Autodesk Inventor part; units mm, degrees
ref_plane "YZ Plane" through (0, 0, 0) normal (1, 0, 0) x (0, 1, 0)
ref_plane "XZ Plane" through (0, 0, 0) normal (0, 1, 0) x (-1, 0, 0)
ref_plane "XY Plane" through (0, 0, 0) normal (0, 0, 1) x (1, 0, 0)
sketch "Sketch1" plane through (0, 0, 0) normal (0, 0, 1) x (1, 0, 0)
  circle A0 centre (0, 3.75) radius 1.75
  line L0 (3.5, -3.25) -> (11.1738, -3.25)
  line L1 (11.1738, -3.25) -> (11.1738, -5.25)
  line L2 (11.1738, -5.25) -> (-11.1738, -5.25)
  line L3 (-11.1738, -5.25) -> (-11.1738, -3.25)
  line L4 (-11.1738, -3.25) -> (-3.5, -3.25)
  line L5 (-3.5, -3.25) -> (-3.5, 3.75)
  arc A1 (3.5, 3.75) -> (-3.5, 3.75) centre (0, 3.75) ccw
  line L6 (3.5, 3.75) -> (3.5, -3.25)
  line L7 (44, 1.75) -> (50, 1.75)
  circle A2 centre (0, 3.75) radius 3.5
  line L8 (0, 3.75) -> (250, 3.75)
  line L9 (50, 1.75) -> (0, 1.75)
  line L10 (0, 1.75) -> (0, 3.75)
  line L11 (0, 3.75) -> (50, 3.75)
  line L12 (50, 3.75) -> (50, 1.75)
  line L13 (50, 1.75) -> (250, 1.75)
  line L14 (250, 1.75) -> (250, 3.75)
  line L15 (250, 3.75) -> (50, 3.75)
  line L16 (50, 3.75) -> (50, 1.75)
  line L17 (0, 1.75) -> (250, 1.75)
  line L18 (250, 1.75) -> (250, 5.75)
  line L19 (250, 5.75) -> (0, 5.75)
  line L20 (0, 5.75) -> (0, 1.75)
  circle A3 centre (0, 3.75) radius 3.5
  point P0 (0, 0)
  point P1 (2.8723, 1.75)
  point P2 (2.8723, 5.75)
  dimension "d0" = 250
  dimension "d1" = 2
extrude "Extrusion1" add sketch "Sketch1" along normal blind 2 contours L8 A2 L9 L10 A0 | A0 L20 L19 A1 L8 | A0 L10 L9 A2 A1 L19 L20 | L8 L12 L7 L9 L6 | L6 L9 A2 | A1 L19 L18 L8 | L8 L14 L13 L12
sketch "Sketch2" plane through (0, 0, 2) normal (0, 0, 1) x (1, 0, 0)
  line L0 (13, -15.35) -> (13, -12.35)
  line L1 (13, -12.35) -> (14.6, -12.35)
  line L2 (14.6, -12.35) -> (14.6, -15.35)
  line L3 (14.6, -15.35) -> (13, -15.35)
  line L4 (15, -16.35) -> (12.5, -16.35)
  line L5 (15, -8.75) -> (15, -16.35)
  line L6 (15, -8.75) -> (15, -5.25)
  line L7 (12.5, -5.25) -> (15, -5.25)
  line L8 (12.5, -16.35) -> (12.5, -5.25)
  line L9 (44, -8.25) -> (41.5181, -8.25)
  line L10 (44, -9.25) -> (46.5, -9.25)
  line L11 (13.75, -5.25) -> (13.75, 7.3756)
  line L12 (44, -8.25) -> (44, 8.5683)
  line L13 (2.8723, 1.75) -> (250, 1.75)
  line L14 (250, 1.75) -> (250, 5.75)
  line L15 (250, 5.75) -> (2.8723, 5.75)
  arc A0 (2.8723, 5.75) -> (2.8723, 1.75) centre (0, 3.75) ccw
  circle A1 centre (0, 3.75) radius 1.75
  line L16 (250, 5.75) -> (2.8723, 5.75)
  line L17 (13.75, 5.75) -> (13.75, 1.75)
  circle A2 centre (13.75, 3.75) radius 0.5
  line L18 (44, 5.75) -> (44, 1.75)
  line L19 (2.8723, 1.75) -> (250, 1.75)
  circle A3 centre (44, 3.75) radius 0.5
  point P0 (0, 0)
  dimension "d4" = 1
  dimension "d5" = 1
extrude "Extrusion2" cut sketch "Sketch2" against normal blind 2 contours A2 L11 | L11 A2 | A3 L12 | L12 A3
sketch "Sketch3" plane through (0, 0, 2) normal (0, 0, 1) x (1, 0, 0)
  line L0 (50, -24.1664) -> (50, 13.5237)
  circle A0 centre (44, 3.75) radius 0.5
  circle A1 centre (13.75, 3.75) radius 0.5
  line L1 (2.8723, 1.75) -> (250, 1.75)
  line L2 (250, 1.75) -> (250, 5.75)
  line L3 (250, 5.75) -> (2.8723, 5.75)
  arc A2 (2.8723, 5.75) -> (2.8723, 1.75) centre (0, 3.75) ccw
  circle A3 centre (0, 3.75) radius 1.75
  line L4 (-50, -43.45) -> (50, -43.45)
  line L5 (250, 5.75) -> (57.9443, 5.75)
  line L6 (57.9443, 5.75) -> (57.9443, -37.1171)
  line L7 (57.9443, -37.1171) -> (250, -37.1171)
  line L8 (250, -37.1171) -> (250, 5.75)
  point P0 (0, 0)
  point P1 (57.9443, 5.75)
extrude "Extrusion3" add sketch "Sketch3" along normal blind 0.5 contours L6 L3 L2 L1 | L1 L8 L7 L6
sketch "Sketch4" plane through (0, 0, 2.5) normal (0, 0, 1) x (1, 0, 0)
  line L0 (250, -37.1171) -> (250, 5.75)
  line L1 (250, 5.75) -> (57.9443, 5.75)
  line L2 (57.9443, 5.75) -> (57.9443, -37.1171)
  line L3 (57.9443, -37.1171) -> (250, -37.1171)
  line L4 (250, -37.1171) -> (250, 1.75)
  line L5 (250, -37.1171) -> (210, -37.1171)
  line L6 (210, -37.1171) -> (210, 5.75)
  line L7 (210, 5.75) -> (250, 5.75)
  line L8 (250, 5.75) -> (250, -37.1171)
  point P0 (0, 0)
  dimension "d10" = 40
extrude "Extrusion4" cut sketch "Sketch4" against normal through all contours L3 L6 L1 L0
sketch "Sketch5" plane through (0, 0, 2) normal (0, 0, 1) x (1, 0, 0)
  line L0 (57.9443, 1.75) -> (57.9443, 5.75)
  line L1 (57.9443, 5.75) -> (2.8723, 5.75)
  arc A0 (2.8723, 5.75) -> (2.8723, 1.75) centre (0, 3.75) ccw
  line L2 (2.8723, 1.75) -> (57.9443, 1.75)
  circle A1 centre (44, 3.75) radius 0.5
  circle A2 centre (13.75, 3.75) radius 0.5
  circle A3 centre (0, 3.75) radius 1.75
  arc A4 (2.8723, 5.75) -> (2.8723, 1.75) centre (0, 3.75) ccw
  line L3 (0, 0.25) -> (7.7599, 0.25)
  line L4 (8.6265, 0.4475) -> (11.3354, 1.75)
  line L5 (2.8723, 1.75) -> (57.9443, 1.75)
  arc A5 (7.7599, 0.25) -> (8.6265, 0.4475) centre (7.7599, 2.25) ccw
  line L6 (0, 3.75) -> (10.3738, 3.75)
  line L7 (0, 7.25) -> (7.7599, 7.25)
  line L8 (8.6265, 7.0525) -> (11.3354, 5.75)
  arc A6 (8.6265, 7.0525) -> (7.7599, 7.25) centre (7.7599, 5.25) ccw
  point P0 (0, 0)
  dimension "d13" = 2
extrude "Extrusion5" add sketch "Sketch5" against normal up to surface (2 mm away) contours L4 A5 L3 A0 L2 | L1 A0 L7 A6 L8
properties part number "wachlarz_1"
Input: part model. Units: mm. Frame: model coordinates. A direction names the side the tool comes from. Give positions to 0.01 mm unless a question says otherwise; leave off trailing zeros. Order: outer loops, then holes, each group sorted by start corner. A loop starts at its lowest first (then second) coordinate and runs counter-clockwise, first axis right, second up. Notation, with made-up numbers: (65.25, -4) - (111.25, -4) arc R9 cw to (111.25, 4) - close; hole circle Ø11 at (-4, 63). An arc over 180 degrees is marked (long way). Answer as a JSON object with one key per item and string values. Group by question number.
Q1. First-contact query: pin 1 Ø8 at (x, y) = (183, -29) entering from -Z; pin 2 Ø7.5 at (x, y) = (21, 2.5) entering from +Z. Flat tips, straight axial feed; report the tip coordinate or a pass-through.
Q2. Set-up query: faces 1 (the face through (133, -15, 2.5)), 2 (the face through (27, 4, 2)). Return all of +Z, -Z, +X, -X, +Y, -Y with unobstructed straight access to the full face (end or side cutting, diameter ignored); none if empty.
Q3. Cut plane C-C, the plane y = -18.5. Output: boundary loops of the cut face in (x, z), then the cut area to 3 significant figures.
Q4. Mould query, pull axis X, two halves, no side actions, for faces 3 (the face through (-3.5, 3.7, 1)), 4 (the face through (133, -17, 2)), 5 (the face through (-0.38, 5.46, 0.99)). Classes: pulls with the +X half, pulls with the -X half, needs draft (parallel to the pull), parting line crosses it, or undercut.
Q5. Line query: probe 1 along X at (y, z) = (3.75, 0.6); probe 2 along Y at (x, z) = (13.75, 0.9); probe 3 along Y at (x, z) = (0, 1.2). Output: solid intervals per line, ascending.
Q6. Cut plane A-A, the plane z = 0.75. Output: boundary loops of the cut face in (x, y).
Q7. Cut plane B-B, the plane x = 70. Output: boundary loops of the cut face in (y, z).
Q8. Cut plane D-D, the plane x = 16.5. Output: boundary loops of the cut face in (y, z), then the cut area to 3 significant figures.
Results:
{
 "1": {"pin 1": "z = 2", "pin 2": "z = 2"},
 "2": {"face 1": "+Z, +X, -X, +Y, -Y", "face 2": "+Z, -X, +Y, -Y"},
 "3": {"outline": "(57.94, 2) - (210, 2) - (210, 2.5) - (57.94, 2.5) - close", "area": "76.0 mm^2"},
 "4": {"face 3": "pulls with the -X half", "face 4": "needs draft", "face 5": "undercut"},
 "5": {"probe 1": "-3.5 to -1.75, 1.75 to 13.25, 14.25 to 43.5, 44.5 to 210", "probe 2": "1.75 to 3.25, 4.25 to 5.75", "probe 3": "0.25 to 2, 5.5 to 7.25"},
 "6": {"outline": "(0, 0.25) - (7.76, 0.25) arc R2 ccw to (8.63, 0.45) - (11.34, 1.75) - (210, 1.75) - (210, 5.75) - (11.34, 5.75) - (8.63, 7.05) arc R2 ccw to (7.76, 7.25) - (0, 7.25) arc R3.5 ccw to start; hole circle Ø3.5 at (0, 3.75); hole circle Ø1 at (13.75, 3.75); hole circle Ø1 at (44, 3.75)"},
 "7": {"outline": "(-37.12, 2) - (1.75, 2) - (1.75, 0) - (5.75, 0) - (5.75, 2.5) - (-37.12, 2.5) - close"},
 "8": {"outline": "(1.75, 0) - (5.75, 0) - (5.75, 2) - (1.75, 2) - close", "area": "8.00 mm^2"}
}
